Model file for the job. Use its own axes, mm. Face numbers are marked on the shaded views. A direction names the side the tool comes from. Give positions to 0.01 mm unless a question says otherwise; leave off trailing zeros. Loops run counter-clockwise (first coordinate to the right, second up) from the corner with the lowest first, then second, coordinate; pieces in that order, holes last. Notation, with made-up numbers: (-32.5, 58.25) -> (-7.5, 58.25) arc R21 ccw to (-7.5, 77.25) -> close; hole circle Ø11 at (13, 16). An arc over 180 degrees is marked (long way). Use CSV: the item, a comma, the result in double quotes. Start each with the question number.
(1) Flat gauge pins, fed straight in: pin 1 (3 mm diameter, centred on x = -3.5, z = 4.5, fed in from -Y); pin 2 (5 mm diameter, centred on x = -5.5, y = 8, fed in from +Z); pin 3 (0.5 mm diameter, centred on y = 7.5, z = 0.5, fed in from +X); pin 4 (8 mm diameter, centred on x = 1, y = 8, fed in from -Z). Where does each tip first touch, or does it go through?
(2) Cut at A-A on z = 5.5. Write the cut outline in (x, y), then the cut area to 3 significant figures.
(3) Pull direction X, two halves, no side cores. Call the marked faces 1, 2, 3 and 4: pulls with the +X half, pulls with the -X half, needs draft (parallel to the pull), parting line crosses it, or undercut.
(4) Drill centre lines: probe 1 along X at (y, z) = (2.75, 7.5); probe 2 along Y at (x, z) = (1, 1.25); probe 3 along Y at (x, z) = (-16, 0.5). Where is each one in solid material? Low to high.
(5) 3-axis set-ups, long thin cutter, end or side, ignore diameter. For the marked faces 5, 6 and 7: which of +Z, -Z, +X, -X, +Y, -Y reach the whole face in a straight line?
(6) Cut at B-B on z = 8.75. Write the cut outline in (x, y).
(7) Cut at C-C on x = 0. State how many separate pieces and enclosed holes the cut face has, then the cut area to 3 significant figures.
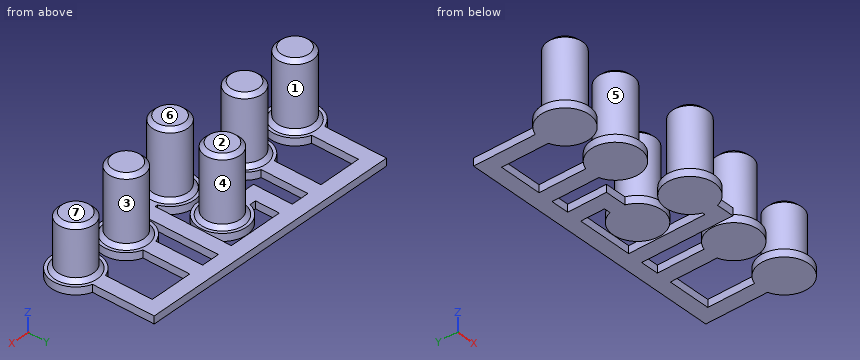
from build123d import *

# Parameters (mm, degrees)
SKIZZE1_R                         = 2.35
AUFSATZ_LINEAR_AUSTRAGEN1_DEPTH   = 10
AUFSATZ_LINEAR_AUSTRAGEN1_2_DEPTH = 10
AUFSATZ_LINEAR_AUSTRAGEN1_3_DEPTH = 10
AUFSATZ_LINEAR_AUSTRAGEN1_4_DEPTH = 10
AUFSATZ_LINEAR_AUSTRAGEN1_5_DEPTH = 10
SKIZZE1_3_R                       = 2.35
AUFSATZ_LINEAR_AUSTRAGEN4_DEPTH   = 8
SKIZZE2_R                         = 3.25
AUFSATZ_LINEAR_AUSTRAGEN2_DEPTH   = 1
AUFSATZ_LINEAR_AUSTRAGEN3_DEPTH   = 1
FASE1_SIZE                        = 0.5
FASE2_SIZE                        = 0.5
FASE3_SIZE                        = 0.5


with BuildPart() as part:
    # Skizze1 → Aufsatz-Linear austragen1 (new body)
    with BuildSketch(Plane.XY):
        with Locations((-17.068817434, 1.838554139)):
            Circle(SKIZZE1_R)
    extrude(amount=AUFSATZ_LINEAR_AUSTRAGEN1_DEPTH)



with BuildPart() as body_2:
    # Skizze1 → Aufsatz-Linear austragen1 2 (new body)
    with BuildSketch(Plane.XY):
        with Locations((-9.321817434, 1.838554139)):
            Circle(SKIZZE1_R)
    extrude(amount=AUFSATZ_LINEAR_AUSTRAGEN1_2_DEPTH)


with BuildPart() as body_3:
    # Skizze1 → Aufsatz-Linear austragen1 3 (new body)
    with BuildSketch(Plane.XY):
        Circle(SKIZZE1_R)
    extrude(amount=AUFSATZ_LINEAR_AUSTRAGEN1_3_DEPTH)


with BuildPart() as body_4:
    # Skizze1 → Aufsatz-Linear austragen1 4 (new body)
    with BuildSketch(Plane.XY):
        with Locations((0.007570249, 6.993531953)):
            Circle(SKIZZE1_R)
    extrude(amount=AUFSATZ_LINEAR_AUSTRAGEN1_4_DEPTH)


with BuildPart() as body_5:
    # Skizze1 → Aufsatz-Linear austragen1 5 (new body)
    with BuildSketch(Plane.XY):
        with Locations((8.839182566, 1.838554139)):
            Circle(SKIZZE1_R)
    extrude(amount=AUFSATZ_LINEAR_AUSTRAGEN1_5_DEPTH)


with BuildPart() as body_6:
    # Skizze1<3> → Aufsatz-Linear austragen4 (new body)
    with BuildSketch(Plane.XY):
        with Locations((16.586182566, 1.838554139)):
            Circle(SKIZZE1_3_R)
    extrude(amount=AUFSATZ_LINEAR_AUSTRAGEN4_DEPTH)


with BuildPart() as part_1:
    add(part.part)

    add(body_2.part)  # Aufsatz-Linear austragen2 merges body 2

    add(body_3.part)  # Aufsatz-Linear austragen2 merges body 3

    add(body_4.part)  # Aufsatz-Linear austragen2 merges body 4

    add(body_5.part)  # Aufsatz-Linear austragen2 merges body 5

    add(body_6.part)  # Aufsatz-Linear austragen2 merges body 6
    # Skizze2 → Aufsatz-Linear austragen2 (add)
    with BuildSketch(Plane.XY):
        with Locations((-17.068817434, 1.838554139)):
            Circle(SKIZZE2_R)
        with Locations((-9.321817434, 1.838554139)):
            Circle(SKIZZE2_R)
        Circle(SKIZZE2_R)
        with Locations((0.007570249, 6.993531953)):
            Circle(SKIZZE2_R)
        with Locations((8.839182566, 1.838554139)):
            Circle(SKIZZE2_R)
        with Locations((16.586182566, 1.838554139)):
            Circle(SKIZZE2_R)
    extrude(amount=AUFSATZ_LINEAR_AUSTRAGEN2_DEPTH)

    # Skizze3 → Aufsatz-Linear austragen3 (add)
    with BuildSketch(Plane.XY):
        Polygon((-18.068817434, 13.164615586), (-18.068817434, 4.930883358), (-16.068817434, 4.930883358), (-16.068817434, 11.164615586), (-10.321817434, 11.164615586), (-10.321817434, 4.930883358), (-8.321817434, 4.930883358), (-8.321817434, 11.164615586), (-5.921817434, 11.164615586), (-5.921817434, 5.993531953), (-3.08475897, 5.993531953), (-3.08475897, 7.993531953), (-3.921817434, 7.993531953), (-3.921817434, 11.164615586), (3.439182566, 11.164615586), (3.439182566, 1), (3.092329219, 1), (3.092329219, -1), (3.439182566, -1), (5.439182566, -1), (5.439182566, 1), (5.439182566, 11.164615586), (7.839182566, 11.164615586), (7.839182566, 4.930883358), (9.839182566, 4.930883358), (9.839182566, 11.164615586), (15.586182566, 11.164615586), (15.586182566, 4.930883358), (17.586182566, 4.930883358), (17.586182566, 13.164615586), align=None)
    extrude(amount=AUFSATZ_LINEAR_AUSTRAGEN3_DEPTH)

    # Fase1
    fase1_edges = [part_1.edges().sort_by_distance(p)[0] for p in [
        (-19.418817434, 1.838554139, 10),
        (-2.35, 0, 10),
        (-2.342429751, 6.993531953, 10),
        (6.489182566, 1.838554139, 10),
        (-11.671817434, 1.838554139, 10),
    ]]
    chamfer(fase1_edges, length=FASE1_SIZE)

    # Fase2
    fase2_edges = [part_1.edges().sort_by_distance(p)[0] for p in [
        (-19.418817434, 1.838554139, 1),
        (-2.35, 0, 1),
        (-2.342429751, 6.993531953, 1),
        (6.489182566, 1.838554139, 1),
        (14.236182566, 1.838554139, 1),
        (-11.671817434, 1.838554139, 1),
    ]]
    chamfer(fase2_edges, length=FASE2_SIZE)

    # Fase3
    fase3_edges = [part_1.edges().sort_by_distance(p)[0] for p in [
        (14.236182566, 1.838554139, 8),
    ]]
    chamfer(fase3_edges, length=FASE3_SIZE)


solid = part_1.part
Check result:
1,pin 1,"y = -1.23"
1,pin 2,"z = 1"
1,pin 3,"x = 17.59"
1,pin 4,"z = 0"
2,outline,"circle Ø4.7 at (-17.07, 1.84); circle Ø4.7 at (-9.32, 1.84); circle Ø4.7 at (0, 0); circle Ø4.7 at (0.01, 6.99); circle Ø4.7 at (8.84, 1.84); circle Ø4.7 at (16.59, 1.84)"
2,area,"104 mm²"
3,face 1,"undercut"
3,face 2,"needs draft"
3,face 3,"undercut"
3,face 4,"parting line crosses it"
4,probe 1,"-19.23 to -14.9, -11.49 to -7.16, 6.67 to 11.01, 14.42 to 18.75"
4,probe 2,"-2.4 to 2.4, 4.59 to 9.4"
4,probe 3,"-1.23 to 4.91, 11.16 to 13.16"
5,face 5,"+Z"
5,face 6,"+Z, +X, -X, +Y, -Y"
5,face 7,"+Z, +X, +Y, -Y"
6,outline,"circle Ø4.7 at (-17.07, 1.84); circle Ø4.7 at (-9.32, 1.84); circle Ø4.7 at (0, 0); circle Ø4.7 at (0.01, 6.99); circle Ø4.7 at (8.84, 1.84)"
7,separate pieces,"3"
7,enclosed holes,"0"
7,area,"99.6 mm²"
